Here's how the part is built. I have some questions about the finished solid (model axes, mm). Coordinates: 2 decimals unless noted, no trailing zeros. Loops run counter-clockwise (first coordinate to the right, second up) from the corner with the lowest first, then second, coordinate; pieces in that order, holes last. Notation, with made-up numbers: M -13,45.25 L 41,45.25 A29 ccw 41,71.25 Z; hole C 42,-21.75 d6. An arc over 180 degrees is marked long. Use one line per item in the form item = value. Start each with the question number.
(1) Imagine slicing it at C-C, the plane z = 1.2. Please give me the cut outline in (x, y).
(2) Imagine slicing it at D-D, the plane x = 33. Please give me the cut outline in (y, z), and give its area (3 significant figures).
(3) Will these pins go through, and if not, where does the flat tip stop? P1, Ø8, axis at x = 0, y = 90, coming from the -Z side; P2, Ø0.8, axis at x = -51, z = 0.5, coming from the +Y side; P3, Ø1.5, axis at y = 74.5, z = 1.5, coming from the -X side.
(4) Imagine slicing it at B-B, the plane y = 21. Please give me the cut outline in (x, z), and give its area (3 significant figures).
(5) Please list where these lines run through material, in increasing order: L1, parallel to Y at x = 0, z = 1.6; L2, parallel to Y at x = -29.5, z = 1.05; L3, parallel to X at y = 89.5, z = 0.85.
(6) Imagine slicing it at A-A, the plane x = 0. Please give me the cut outline in (y, z), and give its area (3 significant figures).
```python
from build123d import *

# Parameters (mm, degrees)
SKIZZE1_R                       = 5
AUFSATZ_LINEAR_AUSTRAGEN1_DEPTH = 2.5


with BuildPart() as part:
    # Skizze1 → Aufsatz-Linear austragen1 (new body)
    with BuildSketch(Plane.XY):
        with BuildLine():
            Line((-65, 0), (65, 0))
            Line((65, 0), (65, 50))
            Line((65, 50), (30, 50))
            ThreePointArc((30, 50), (22.928932188, 52.928932188), (20, 60))
            Line((20, 60), (20, 90))
            ThreePointArc((20, 90), (0, 110), (-20, 90))
            Line((-20, 90), (-20, 60))
            ThreePointArc((-20, 60), (-22.928932188, 52.928932188), (-30, 50))
            Line((-30, 50), (-65, 50))
            Line((-65, 50), (-65, 0))
        make_face()
        with Locations((0, 90)):
            Circle(SKIZZE1_R, mode=Mode.SUBTRACT)
        with BuildLine():
            Line((-30, 27), (30, 27))
            ThreePointArc((30, 27), (36, 21), (30, 15))
            Line((30, 15), (-30, 15))
            ThreePointArc((-30, 15), (-36, 21), (-30, 27))
        make_face(mode=Mode.SUBTRACT)
    extrude(amount=AUFSATZ_LINEAR_AUSTRAGEN1_DEPTH)


solid = part.part
```
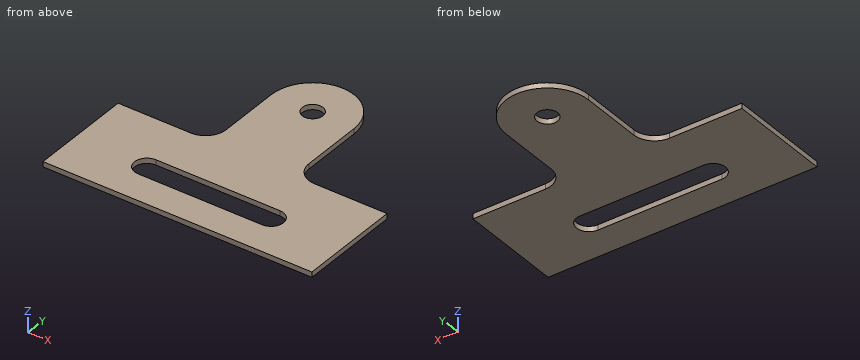
Answer:
q1.outline = M -65,0 L 65,0 L 65,50 L 30,50 A10 cw 20,60 L 20,90 A20 ccw -20,90 L -20,60 A10 cw -30,50 L -65,50 Z; hole M -30,15 L 30,15 A6 ccw 30,27 L -30,27 A6 ccw Z; hole C 0,90 d10
q2.outline = M 0,0 L 15.8,0 L 15.8,2.5 L 0,2.5 Z; M 26.2,0 L 50,0 L 50,2.5 L 26.2,2.5 Z
q2.area = 99.0 mm²
q3.P1 = through
q3.P2 = 50
q3.P3 = -20
q4.outline = M -65,0 L -36,0 L -36,2.5 L -65,2.5 Z; M 36,0 L 65,0 L 65,2.5 L 36,2.5 Z
q4.area = 145 mm²
q5.L1 = 0 to 15, 27 to 85, 95 to 110
q5.L2 = 0 to 15, 27 to 50.01
q5.L3 = -20 to -4.97, 4.97 to 20
q6.outline = M 0,0 L 15,0 L 15,2.5 L 0,2.5 Z; M 27,0 L 85,0 L 85,2.5 L 27,2.5 Z; M 95,0 L 110,0 L 110,2.5 L 95,2.5 Z
q6.area = 220 mm²
